```python
from build123d import *

# Parameters (mm, degrees)
BOSS_EXTRUDE1_DEPTH = 20
CUT_EXTRUDE1_DEPTH  = 24.053894737


with BuildPart() as part:
    # Sketch1 → Boss-Extrude1 (new body)
    with BuildSketch(Plane.XY):
        Polygon((-20.053894737, 23), (0, 0), (3, 0), (3, 35), (-20.053894737, 35), align=None)
    extrude(amount=BOSS_EXTRUDE1_DEPTH)

    # Sketch2 → Cut-Extrude1 (cut, through all)
    with BuildSketch(Plane(origin=(3, 0, 0), x_dir=(0, 0, -1), z_dir=(1, 0, 0))):
        Polygon((-5, 33), (-5, 35), (-16, 35), (-16, 33), (-18, 33), (-18, 30), (-3, 30), (-3, 33), align=None)
    extrude(amount=-CUT_EXTRUDE1_DEPTH, mode=Mode.SUBTRACT)


solid = part.part
```
Geometry: final body of the model. Coordinates: model frame, mm. A direction names the side the tool comes from. Give positions to 0.01 mm unless a question says otherwise; leave off trailing zeros. Order: outer loops, then holes, each group sorted by start corner. A loop starts at its lowest first (then second) coordinate and runs counter-clockwise, first axis right, second up. Notation, with made-up numbers: (-3, 41.25) -> (28, 41.25) arc R25 cw to (28, 61.25) -> close; hole circle Ø8 at (81, -19.5). An arc over 180 degrees is marked (long way). Write each question's results on one line, items separated by ' | '. Start each with the question number.
1) Section C-C (z = 7.25). Return loops of the section in (x, y), then the cut area to 3 significant figures.
2) Section B-B (x = 0.5). Return loops of the section in (y, z).
3) Section A-A (z = 3.75). Return loops of the section in (x, y).
4) Draft query along Y for faces 1 (the flat face through (-8, 35, 2)), 2 (the flat face through (-8, 33, 17)), 3 (the flat face through (-8, 34, 16)), 4 (the flat face through (-8, 31, 3)). Return one class per face: pulls with the +Y half, pulls with the -Y half, needs draft (parallel to the pull), parting line crosses it, or undercut.
5) Set-up query: faces 5 (the flat face through (-20.054, 28, 10)), 6 (the flat face through (-8, 33, 4)), 7 (the flat face through (-8, 34, 5)). Return all of +Z, -Z, +X, -X, +Y, -Y with unobstructed straight access to the full face (end or side cutting, diameter ignored); none if empty.
6) Section D-D (y = 12.5). Return loops of the section in (x, z).
7) First-contact query: pin 1 (3 mm diameter, centred on y = 21, z = 8, fed in from -X); pin 2 (3 mm diameter, centred on x = -7, z = 3.5, fed in from -Y); pin 3 (12 mm diameter, centred on y = 4.5, z = 16.5, fed in from -X). Flat tips, straight axial feed; report the tip coordinate or a pass-through.
8) Line query: line 1 (Z direction, x = -2.25, y = 32); line 2 (Y direction, x = 1.5, z = 14.75); line 3 (Y direction, x = -8, z = 3.25). Output: solid intervals per line, ascending. Write a range as from..to.
Calculated:
1) outline: (-20.05, 23) -> (0, 0) -> (3, 0) -> (3, 30) -> (-20.05, 30) -> close | area: 461 mm2
2) outline: (0, 0) -> (35, 0) -> (35, 5) -> (33, 5) -> (33, 3) -> (30, 3) -> (30, 18) -> (33, 18) -> (33, 16) -> (35, 16) -> (35, 20) -> (0, 20) -> close
3) outline: (-20.05, 23) -> (0, 0) -> (3, 0) -> (3, 30) -> (-20.05, 30) -> close; (-20.05, 33) -> (3, 33) -> (3, 35) -> (-20.05, 35) -> close
4) face 1: pulls with the +Y half | face 2: undercut | face 3: needs draft | face 4: undercut
5) face 5: +Z, -Z, -X, +Y, -Y | face 6: +X, -X | face 7: +X, -X, +Y
6) outline: (-10.9, 0) -> (3, 0) -> (3, 20) -> (-10.9, 20) -> close
7) pin 1: x = -19.62 | pin 2: y = 6.31 | pin 3: x = -9.16
8) line 1: 0..3, 18..20 | line 2: 0..30 | line 3: 9.18..30, 33..35
